from build123d import *

# Parameters (mm, degrees)
SKETCH003_W     = 44
SKETCH003_H     = 20
PAD001_DEPTH    = 17
SKETCH_R        = 26
PAD_DEPTH       = 29
SKETCH001_R     = 25.1
POCKET_DEPTH    = 2
SKETCH002_R     = 24.5
POCKET001_DEPTH = 26


with BuildPart() as pad001:
    # Sketch003 → Pad001 (new body)
    with BuildSketch(Plane.XY.offset(12)):
        with Locations((0, -17)):
            Rectangle(SKETCH003_W, SKETCH003_H)
    extrude(amount=PAD001_DEPTH)


with BuildPart() as cut:
    # Sketch → Pad (new body)
    with BuildSketch(Plane.XY):
        Circle(SKETCH_R)
    extrude(amount=PAD_DEPTH)

    # Sketch001 → Pocket (cut)
    with BuildSketch(Plane.XY.offset(29)):
        Circle(SKETCH001_R)
    extrude(amount=-POCKET_DEPTH, mode=Mode.SUBTRACT)

    # Sketch002 → Pocket001 (cut)
    with BuildSketch(Plane.XY.offset(27)):
        Circle(SKETCH002_R)
    extrude(amount=-POCKET001_DEPTH, mode=Mode.SUBTRACT)

    # Cut: cut Pad001
    add(pad001.part, mode=Mode.SUBTRACT)


solid = cut.part
Input: part model. Units: mm. Frame: model coordinates. A direction names the side the tool comes from. Give positions to 0.01 mm unless a question says otherwise; leave off trailing zeros. Loops run counter-clockwise (first coordinate to the right, second up) from the corner with the lowest first, then second, coordinate; pieces in that order, holes last. Notation, with made-up numbers: M 22.5,68 L 38.5,68 A27 ccw 38.5,102 Z; hole C -20.75,6 d8. An arc over 180 degrees is marked long. Use CSV: the item, a comma, the result in double quotes.
(1) Section B-B, the plane y = 0. Return loops of the section in (x, z).
Outcome:
outline,"M -26,0 L 26,0 L 26,29 L 25.1,29 L 25.1,27 L 24.5,27 L 24.5,1 L -24.5,1 L -24.5,27 L -25.1,27 L -25.1,29 L -26,29 Z"
(2) Section C-C, the plane z = 13.75. Return loops of the section in (x, y), plus the area to 3 significant figures.
Outcome:
outline,"M -22,-13.86 L -22,-10.78 A24.5 cw long 22,-10.78 L 22,-13.86 A26 ccw long Z"
area,"158 mm²"
(3) Pin query (flat end, axial travel): P1, Ø12, axis at x = -18, z = 25, coming from the -Y side; P2, Ø10, axis at y = 13, z = 19, coming from the +X side; P3, Ø0.9, axis at y = -12.5, z = 18.5, coming from the -X side; P4, Ø10, axis at x = -10.5, y = 3, coming from the -Z side. Return the tip coordinate at first contact, or that it passes through.
Outcome:
P1,"stops at y = -13.86"
P2,"stops at x = 24.74"
P3,"stops at x = -23.04"
P4,"stops at z = 0"
(4) Section D-D, the plane z = 10. Return loops of the section in (x, y), plus the area to 3 significant figures.
Outcome:
outline,"C 0,0 d52; hole C 0,0 d49"
area,"238 mm²"
(5) Set-up query: faces 5 (the face through (-22, -12, 20)), 6 (the face through (-3.8, 24.5, 27)), 7 (the face through (0, 0, 0)). Return all of +Z, -Z, +X, -X, +Y, -Y with unobstructed straight access to the full face (end or side cutting, diameter ignored); none if empty.
Outcome:
face 5,"+Z, -Y"
face 6,"+Z"
face 7,"-Z, +X, -X, +Y, -Y"
(6) Material intervals for L1, parallel to X at y = 0, z = 27.9; L2, parallel to Z at x = -13.5, y = 1; L3, parallel to X at y = -3, z = 27.5, sorted ascending. Write a range as [from, to].
Outcome:
L1,"x = [-26, -25.1], [25.1, 26]"
L2,"z = [0, 1]"
L3,"x = [-25.83, -24.92], [24.92, 25.83]"
(7) Pull-direction query (X, two-part tool) for faces 1 (the face through (-3.38, 25.78, 14.3)), 2 (the face through (13.17, 20.66, 14.18)), 3 (the face through (-8, 24, 29)), 4 (the face through (22, -12, 20)); classes: pulls with the +X half, pulls with the -X half, needs draft (parallel to the pull), parting line crosses it, or undercut.
Outcome:
face 1,"parting line crosses it"
face 2,"undercut"
face 3,"needs draft"
face 4,"undercut"
(8) Section A-A, the plane x = 0. Return loops of the section in (y, z), plus the area to 3 significant figures.
Outcome:
outline,"M -26,0 L 26,0 L 26,29 L 25.1,29 L 25.1,27 L 24.5,27 L 24.5,1 L -24.5,1 L -24.5,12 L -26,12 Z"
area,"109 mm²"
